The drawing under review shows one solid part. Ordinate dimensions are in mm from its lowest x, y, z. A direction names the side the tool comes from. Give positions to 0.01 mm unless a question says otherwise; leave off trailing zeros. Write each loop counter-clockwise with the first axis right and the second up, starting at its lowest first coordinate (ties: lowest second). Pieces come first, ordered by that corner, then holes.
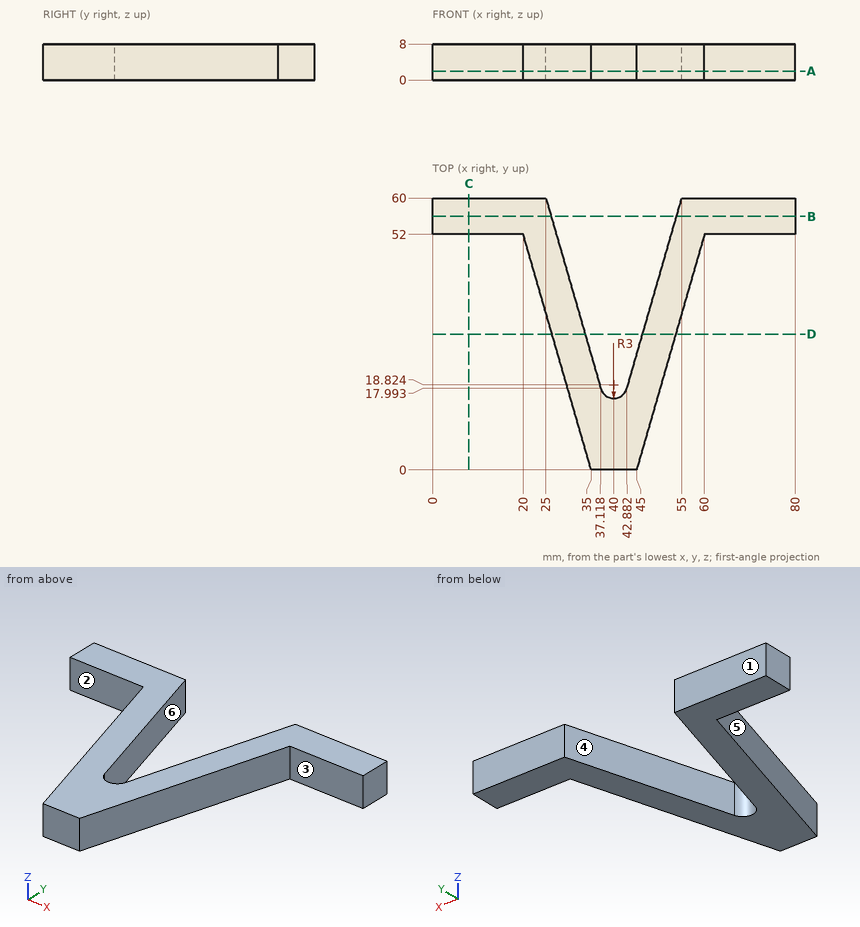
1) Insertion check: pin 1 (2 mm diameter, centred on x = 9.5, z = 1, fed in from -Y); pin 2 (2 mm diameter, centred on y = 18.5, z = 5.5, fed in from -X) (1 decimal); pin 3 (3 mm diameter, centred on y = 39, z = 7, fed in from +X). Each pin has a flat end and moves straight along its axis. Give the tip position at first contact, or say it passes through.
2) Consider section D-D, the plane y = 30. Give the boundary of the cut face in (x, z).
3) Consider section A-A, the plane z = 2. Give the boundary of the cut face in (x, y).
4) Consider section C-C, the plane x = 8. Give the boundary of the cut face in (y, z), then the cut area to 3 significant figures.
5) To check wall thickness, follow probe 1 along Y at (x, z) = (16, 6); probe 2 along X at (y, z) = (41, 5); probe 3 along X at (y, z) = (36.5, 5). State the ranges of each line that lie inside material, in increasing order.
6) Tool access review of the marked faces 1 and 2: name each direction out of +Z, -Z, +X, -X, +Y, -Y from which nothing blocks a thin tool from reaching the whole face with its end or side.
7) Consider section B-B, the plane y = 56. Give the boundary of the cut face in (x, z).
8) The part is to be moulded in two halves that separate along X. For the marked faces 3, 4, 5 and 6, say which applies: +X half, -X half, draft (parallel to the pull), parting line (faces both ways), or undercut.
Answer block:
1. pin 1: stops at y = 52
1. pin 2: stops at x = 29.4
1. pin 3: stops at x = 56.68
2. outline: (26.35, 0) - (33.65, 0) - (33.65, 8) - (26.35, 8) - close; (46.35, 0) - (53.65, 0) - (53.65, 8) - (46.35, 8) - close
3. outline: (0, 52) - (20, 52) - (35, 0) - (45, 0) - (60, 52) - (80, 52) - (80, 60) - (55, 60) - (42.88, 17.99) arc R3 cw to (37.12, 17.99) - (25, 60) - (0, 60) - close
4. outline: (52, 0) - (60, 0) - (60, 8) - (52, 8) - close
4. area: 64.0 mm2
5. probe 1: y = 52 to 60
5. probe 2: x = 23.17 to 30.48, 49.52 to 56.83
5. probe 3: x = 24.47 to 31.78, 48.22 to 55.53
6. face 1: +Z, -Z, +X, -X, +Y
6. face 2: +Z, -Z, -X, -Y
7. outline: (0, 0) - (26.15, 0) - (26.15, 8) - (0, 8) - close; (53.85, 0) - (80, 0) - (80, 8) - (53.85, 8) - close
8. face 3: draft
8. face 4: undercut
8. face 5: -X half
8. face 6: undercut
